The model under review builds one solid part; all positions refer to its coordinate system, in mm. Face numbers are marked on the shaded views. A direction names the side the tool comes from. Give positions to 0.01 mm unless a question says otherwise; leave off trailing zeros. Order: outer loops, then holes, each group sorted by start corner. A loop starts at its lowest first (then second) coordinate and runs counter-clockwise, first axis right, second up. Notation, with made-up numbers: (-12.5, 77) - (40.5, 77) arc R17 cw to (40.5, 94) - close; hole circle Ø4 at (10.25, 13). An arc over 180 degrees is marked (long way). Use CSV: the item, a comma, the result in double quotes.
```python
from build123d import *

# Parameters (mm, degrees)
BASE_FLANGE1_DEPTH = 100
CUT_EXTRUDE1_REACH = 163.496
SKETCH6_R          = 8.5
CUT_EXTRUDE2_REACH = 124.348
SKETCH7_R          = 3
FILLET1_R          = 5


# Sheet-metal steps are written as plain solids
with BuildPart() as part:
    # Sketch1 → Base-Flange1 (new body)
    with BuildSketch(Plane.XY):
        with BuildLine():
            Line((-60, 41), (-60, 8))
            ThreePointArc((-60, 8), (-57.656854249, 2.343145751), (-52, 0))
            Line((-52, 0), (52, 0))
            ThreePointArc((52, 0), (57.656854249, 2.343145751), (60, 8))
            Line((60, 8), (60, 41))
            Line((60, 41), (56, 41))
            Line((56, 41), (56, 8))
            ThreePointArc((56, 8), (54.828427125, 5.171572875), (52, 4))
            Line((52, 4), (-52, 4))
            ThreePointArc((-52, 4), (-54.828427125, 5.171572875), (-56, 8))
            Line((-56, 8), (-56, 41))
            Line((-56, 41), (-60, 41))
        make_face()
    extrude(amount=BASE_FLANGE1_DEPTH)

    # Cut-Extrude1: up to this face of the body (flat: up to its plane)
    cut_extrude1_end = Plane(part.part.faces().sort_by_distance((-60, 24.5, 50))[0])
    # Sketch6 → Cut-Extrude1 (cut, up to the picked face)
    with BuildSketch(Plane(origin=(60, 0, 0), x_dir=(0, 0, -1), z_dir=(1, 0, 0)), mode=Mode.PRIVATE) as cut_extrude1_sk1:
        with Locations((-50, 25.4)):
            Circle(SKETCH6_R)
    cut_extrude1_tool1 = split(extrude(cut_extrude1_sk1.sketch, amount=-CUT_EXTRUDE1_REACH, mode=Mode.PRIVATE), bisect_by=cut_extrude1_end, keep=Keep.BOTH, mode=Mode.PRIVATE)
    add(cut_extrude1_tool1.solids().sort_by(Axis((60, 25.4, 50), (-1, 0, 0)))[0], mode=Mode.SUBTRACT)

    # Sketch7 → Cut-Extrude2 (cut, up to next)
    with BuildSketch(Plane(origin=(0, 4, 0), x_dir=(1, 0, 0), z_dir=(0, 1, 0)), mode=Mode.PRIVATE) as cut_extrude2_sk1:
        with Locations(Location((-43, -11.1, 0), (0, 0, 270))):
            Circle(SKETCH7_R)
    cut_extrude2_tool1 = extrude(cut_extrude2_sk1.sketch, amount=-CUT_EXTRUDE2_REACH, mode=Mode.PRIVATE) & part.part
    # Sketch7 → Cut-Extrude2 (cut, up to next)
    with BuildSketch(Plane(origin=(0, 4, 0), x_dir=(1, 0, 0), z_dir=(0, 1, 0)), mode=Mode.PRIVATE) as cut_extrude2_sk2:
        with Locations(Location((43, -11.1, 0), (0, 0, 90))):
            Circle(SKETCH7_R)
    cut_extrude2_tool2 = extrude(cut_extrude2_sk2.sketch, amount=-CUT_EXTRUDE2_REACH, mode=Mode.PRIVATE) & part.part
    # Sketch7 → Cut-Extrude2 (cut, up to next)
    with BuildSketch(Plane(origin=(0, 4, 0), x_dir=(1, 0, 0), z_dir=(0, 1, 0)), mode=Mode.PRIVATE) as cut_extrude2_sk3:
        with Locations(Location((-43, -88.9, 0), (0, 0, 90))):
            Circle(SKETCH7_R)
    cut_extrude2_tool3 = extrude(cut_extrude2_sk3.sketch, amount=-CUT_EXTRUDE2_REACH, mode=Mode.PRIVATE) & part.part
    # Sketch7 → Cut-Extrude2 (cut, up to next)
    with BuildSketch(Plane(origin=(0, 4, 0), x_dir=(1, 0, 0), z_dir=(0, 1, 0)), mode=Mode.PRIVATE) as cut_extrude2_sk4:
        with Locations(Location((43, -88.9, 0), (0, 0, 270))):
            Circle(SKETCH7_R)
    cut_extrude2_tool4 = extrude(cut_extrude2_sk4.sketch, amount=-CUT_EXTRUDE2_REACH, mode=Mode.PRIVATE) & part.part
    # Sketch7 → Cut-Extrude2 (cut, up to next)
    with BuildSketch(Plane(origin=(0, 4, 0), x_dir=(1, 0, 0), z_dir=(0, 1, 0)), mode=Mode.PRIVATE) as cut_extrude2_sk5:
        with BuildLine():
            Line((-35.5, -67.5), (35.5, -67.5))
            ThreePointArc((35.5, -67.5), (37.621320344, -66.621320344), (38.5, -64.5))
            Line((38.5, -64.5), (38.5, -35.5))
            ThreePointArc((38.5, -35.5), (37.621320344, -33.378679656), (35.5, -32.5))
            Line((35.5, -32.5), (-35.5, -32.5))
            ThreePointArc((-35.5, -32.5), (-37.621320344, -33.378679656), (-38.5, -35.5))
            Line((-38.5, -35.5), (-38.5, -64.5))
            ThreePointArc((-38.5, -64.5), (-37.621320344, -66.621320344), (-35.5, -67.5))
        make_face()
    cut_extrude2_tool5 = extrude(cut_extrude2_sk5.sketch, amount=-CUT_EXTRUDE2_REACH, mode=Mode.PRIVATE) & part.part
    add(cut_extrude2_tool1.solids().sort_by_distance((-43, 4, 11.1))[0], mode=Mode.SUBTRACT)
    add(cut_extrude2_tool2.solids().sort_by_distance((43, 4, 11.1))[0], mode=Mode.SUBTRACT)
    add(cut_extrude2_tool3.solids().sort_by_distance((-43, 4, 88.9))[0], mode=Mode.SUBTRACT)
    add(cut_extrude2_tool4.solids().sort_by_distance((43, 4, 88.9))[0], mode=Mode.SUBTRACT)
    add(cut_extrude2_tool5.solids().sort_by_distance((0, 4, 50))[0], mode=Mode.SUBTRACT)

    # Fillet1
    fillet1_edges = [part.edges().sort_by_distance(p)[0] for p in [
        (58, 41, 0),
        (-58, 41, 0),
        (58, 41, 100),
        (-58, 41, 100),
    ]]
    fillet(fillet1_edges, radius=FILLET1_R)


solid = part.part
```
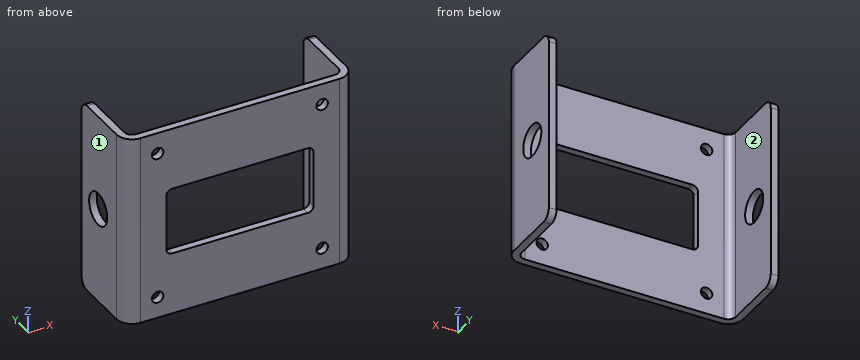
Item 1: Clearance check with flat-ended pins moving along their axes: pin 1 (8 mm diameter, centred on x = 43, z = 88.9, fed in from +Y); pin 2 (1.5 mm diameter, centred on x = 3, z = 15.5, fed in from -Y); pin 3 (5 mm diameter, centred on x = -43, z = 88.9, fed in from +Y); pin 4 (4.5 mm diameter, centred on y = 1, z = 44, fed in from -X). State where each tip first meets the part, or that it passes through.
Results list:
pin 1,"stops at y = 4"
pin 2,"stops at y = 0"
pin 3,"passes through"
pin 4,"stops at x = -58.44"
Item 2: Take a section at A-A, the plane x = 43. Give the boundary of the cut face in (y, z), and give its area (3 significant figures).
Results list:
outline,"(0, 0) - (4, 0) - (4, 8.1) - (0, 8.1) - close; (0, 14.1) - (4, 14.1) - (4, 85.9) - (0, 85.9) - close; (0, 91.9) - (4, 91.9) - (4, 100) - (0, 100) - close"
area,"352 mm2"
Item 3: Take a section at B-B, the plane y = 15.5. Give the boundary of the cut face in (x, z), and give its area (3 significant figures).
Results list:
outline,"(-60, 0) - (-56, 0) - (-56, 100) - (-60, 100) - close; (56, 0) - (60, 0) - (60, 100) - (56, 100) - close"
area,"800 mm2"
Item 4: Take a section at D-D, the plane x = -24. Give the boundary of the cut face in (y, z), and give its area (3 significant figures).
Results list:
outline,"(0, 0) - (4, 0) - (4, 32.5) - (0, 32.5) - close; (0, 67.5) - (4, 67.5) - (4, 100) - (0, 100) - close"
area,"260 mm2"
Item 5: Wall thickness on L1, parallel to X at y = 29, z = 82; L2, parallel to X at y = 1.9, z = 11.1; L3, parallel to X at y = 1.25, z = 11.1: over which ranges is each line inside the solid? List them lowest first.
Results list:
L1,"x = -60 to -56, 56 to 60"
L2,"x = -57.18 to -46, -40 to 40, 46 to 57.18"
L3,"x = -56.29 to -46, -40 to 40, 46 to 56.29"
Item 6: Tool access review of the marked faces 1 and 2: name each direction out of +Z, -Z, +X, -X, +Y, -Y from which nothing blocks a thin tool from reaching the whole face with its end or side.
Results list:
face 1,"+Z, -Z, -X, +Y, -Y"
face 2,"+Z, -Z, +Y"
Item 7: Take a section at C-C, the plane z = 50. Give the boundary of the cut face in (x, y), and give its area (3 significant figures).
Results list:
outline,"(-60, 8) arc R8 ccw to (-52, 0) - (-38.5, 0) - (-38.5, 4) - (-52, 4) arc R4 cw to (-56, 8) - (-56, 16.9) - (-60, 16.9) - close; (-60, 33.9) - (-56, 33.9) - (-56, 41) - (-60, 41) - close; (38.5, 0) - (52, 0) arc R8 ccw to (60, 8) - (60, 16.9) - (56, 16.9) - (56, 8) arc R4 cw to (52, 4) - (38.5, 4) - close; (56, 33.9) - (60, 33.9) - (60, 41) - (56, 41) - close"
area,"311 mm2"
